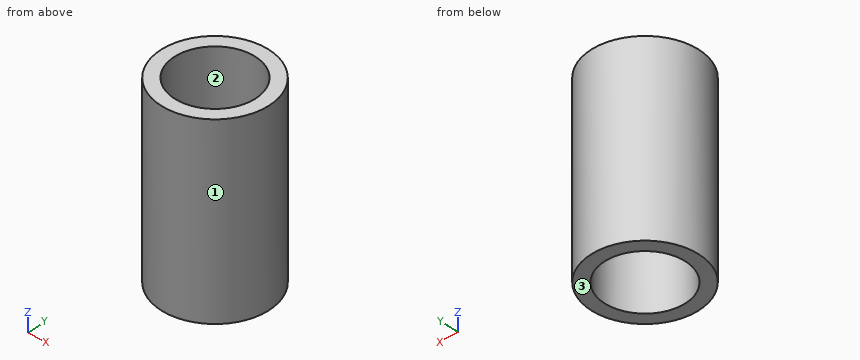
from build123d import *

# Parameters (mm, degrees)
SKETCH1_R          = 12.7
BASE_EXTRUDE_DEPTH = 28.575
SKETCH2_R          = 9.525
CUT_EXTRUDE1_DEPTH = 34.750712955
SKETCH_1_R         = 12.7
SKETCH_1_R_2       = 9.525
EXTRUDE_1_DEPTH    = 43.58


with BuildPart() as part:
    # Sketch1 → Base-Extrude (new body)
    with BuildSketch(Plane.XY):
        Circle(SKETCH1_R)
    extrude(amount=BASE_EXTRUDE_DEPTH)

    # Sketch2 → Cut-Extrude1 (cut, through all)
    with BuildSketch(Plane.XY.offset(28.575)):
        Circle(SKETCH2_R)
    extrude(amount=-CUT_EXTRUDE1_DEPTH, mode=Mode.SUBTRACT)

    # Эскиз1 → Бобышка-Вытянуть1 (add)
    with BuildSketch(Plane.XY.offset(28.575)):
        Circle(SKETCH_1_R)
        Circle(SKETCH_1_R_2, mode=Mode.SUBTRACT)
    extrude(amount=-EXTRUDE_1_DEPTH)


solid = part.part
Could you check a few things on this model? Use its own coordinates, in mm. Face numbers are marked on the shaded views. Give positions to 0.01 mm unless a question says otherwise; leave off trailing zeros. Order: outer loops, then holes, each group sorted by start corner. A loop starts at its lowest first (then second) coordinate and runs counter-clockwise, first axis right, second up.
Item 1: I need wall thicknesses on line 1 (Y direction, x = 0, z = 2.5) (3 decimals); line 2 (X direction, y = -8.75, z = -11); line 3 (Y direction, x = 1.25, z = -2). Which ranges of each line are inside material? Lowest first, please.
Item 2: If we section it at C-C, the plane z = 15: Write out the boundary of the cut face in (x, y) (3 decimals), plus the area to 3 significant figures.
Item 3: If we section it at D-D, the plane y = -10.75: Write out the boundary of the cut face in (x, z) (3 decimals).
Item 4: I'm going to push flat-ended pins straight in: pin 1 (5 mm diameter, centred on y = -0.5, z = 3, fed in from -X); pin 2 (1.5 mm diameter, centred on x = -7.5, z = 7.5, fed in from -Y); pin 3 (4 mm diameter, centred on y = -10, z = 14.5, fed in from -X); pin 4 (12 mm diameter, centred on x = 6.5, z = 2.5, fed in from +Y). Where does each tip first touch, or does it pass through?
Item 5: If we section it at A-A, the plane x = 0: Write out the boundary of the cut face in (y, z) (3 decimals).
Item 6: If we mould it in two halves opening along Y, with no side actions, what happens to the marked faces 1, 2 and 3? For each: pulls with the +Y half, pulls with the -Y half, needs draft (parallel to the pull), parting line crosses it, or undercut.
Values:
1. line 1: y = -12.7 to -9.525, 9.525 to 12.7
1. line 2: x = -9.2 to -3.76, 3.76 to 9.2
1. line 3: y = -12.64 to -9.44, 9.44 to 12.64
2. outline: circle Ø25.4 at (0, 0); hole circle Ø19.05 at (0, 0)
2. area: 222 mm2
3. outline: (-6.762, -15.005) - (6.762, -15.005) - (6.762, 28.575) - (-6.762, 28.575) - close
4. pin 1: stops at x = -12.7
4. pin 2: stops at y = -10.76
4. pin 3: stops at x = -9.86
4. pin 4: stops at y = 12.69
5. outline: (-12.7, -15.005) - (-9.525, -15.005) - (-9.525, 28.575) - (-12.7, 28.575) - close; (9.525, -15.005) - (12.7, -15.005) - (12.7, 28.575) - (9.525, 28.575) - close
6. face 1: parting line crosses it
6. face 2: undercut
6. face 3: needs draft
